```python
from build123d import *

# Parameters (mm, degrees)
SKETCH1_R           = 30.625
SKETCH1_R_2         = 12
BOSS_EXTRUDE1_DEPTH = 4.22
SKETCH1_4_R         = 52.5
SKETCH1_4_R_2       = 45
SKETCH1_4_R_3       = 30.625
BOSS_EXTRUDE2_DEPTH = 2
SKETCH2_R           = 1.5
CUT_EXTRUDE1_DEPTH  = 20


with BuildPart() as part:
    # Sketch1 → Boss-Extrude1 (new body)
    with BuildSketch(Plane.XY):
        Circle(SKETCH1_R)
        Circle(SKETCH1_R_2, mode=Mode.SUBTRACT)
    extrude(amount=-BOSS_EXTRUDE1_DEPTH)

    # Sketch1_4 → Boss-Extrude2 (add)
    # profile 1 of 2: a face of its own
    with BuildSketch(Plane.XY):
        Circle(SKETCH1_4_R)
        Circle(SKETCH1_4_R_2, mode=Mode.SUBTRACT)
    # profile 2 of 2: a face of its own
    with BuildSketch(Plane.XY):
        Circle(SKETCH1_4_R_2)
        Circle(SKETCH1_4_R_3, mode=Mode.SUBTRACT)
    extrude(amount=-BOSS_EXTRUDE2_DEPTH)

    # Sketch2 → Cut-Extrude1 (cut)
    with BuildSketch(Plane.XY):
        with Locations((-34.471455583, 34.471455583)):
            Circle(SKETCH2_R)
        with Locations((34.471455583, 34.471455583)):
            Circle(SKETCH2_R)
        with Locations((34.471455583, -34.471455583)):
            Circle(SKETCH2_R)
        with Locations((-34.471455583, -34.471455583)):
            Circle(SKETCH2_R)
        with Locations((0, 22.5)):
            Circle(SKETCH2_R)
        with Locations((22.5, 0)):
            Circle(SKETCH2_R)
        with Locations((0, -22.5)):
            Circle(SKETCH2_R)
        with Locations((-22.5, 0)):
            Circle(SKETCH2_R)
    extrude(amount=-CUT_EXTRUDE1_DEPTH, mode=Mode.SUBTRACT)


solid = part.part
```
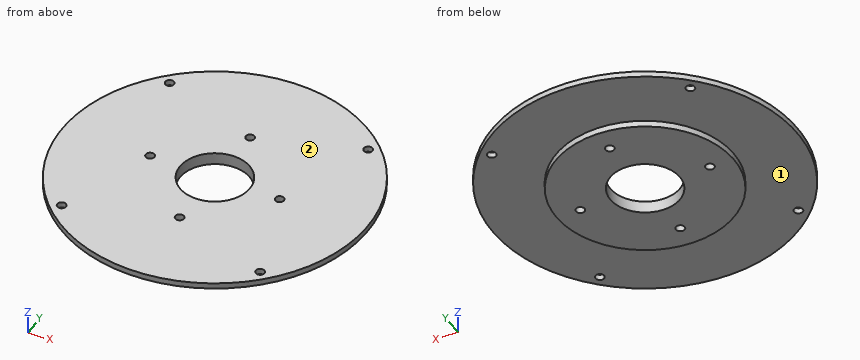
The model under review builds one solid part; all positions refer to its coordinate system, in mm. Face numbers are marked on the shaded views. A direction names the side the tool comes from. Round coordinates to 2 decimals unless told otherwise and drop trailing zeros. Order: outer loops, then holes, each group sorted by start corner. A loop starts at its lowest first (then second) coordinate and runs counter-clockwise, first axis right, second up.
(1) Take a section at C-C, the plane z = -3.3. State the section outline as (x, y) points (3 decimals).
Working result:
outline: circle Ø61.25 at (0, 0); hole circle Ø3 at (-22.5, 0); hole circle Ø24 at (0, 0); hole circle Ø3 at (0, -22.5); hole circle Ø3 at (0, 22.5); hole circle Ø3 at (22.5, 0)
(2) Take a section at A-A, the plane y = 0. State the section outline as (x, z) points (3 decimals), plus the area to 3 significant figures.
Working result:
outline: (-52.5, -2) - (-30.625, -2) - (-30.625, -4.22) - (-24, -4.22) - (-24, 0) - (-52.5, 0) - close; (-21, -4.22) - (-12, -4.22) - (-12, 0) - (-21, 0) - close; (12, -4.22) - (21, -4.22) - (21, 0) - (12, 0) - close; (24, -4.22) - (30.625, -4.22) - (30.625, -2) - (52.5, -2) - (52.5, 0) - (24, 0) - close
area: 219 mm2
(3) Take a section at D-D, the plane x = -22.5. State the section outline as (y, z) points, plus the area to 3 significant figures.
Working result:
outline: (-47.43, -2) - (-20.78, -2) - (-20.78, -4.22) - (-1.5, -4.22) - (-1.5, 0) - (-47.43, 0) - close; (1.5, -4.22) - (20.78, -4.22) - (20.78, -2) - (47.43, -2) - (47.43, 0) - (1.5, 0) - close
area: 269 mm2
(4) For P1, Ø4, axis at x = 34.47, y = 34.47, coming from the -Z side; P2, Ø1, axis at y = 5, z = -3.5, coming from the -X side, all flat-tipped, find the tip position at first contact; note any pin that passes through.
Working result:
P1: stops at z = -2
P2: stops at x = -30.29
(5) Tool access review of the marked faces 1 and 2: name each direction out of +Z, -Z, +X, -X, +Y, -Y from which nothing blocks a thin tool from reaching the whole face with its end or side.
Working result:
face 1: -Z
face 2: +Z, +X, -X, +Y, -Y
(6) Wall thickness on L1, parallel to Y at x = 0, z = -2.3 (3 decimals); L2, parallel to Z at x = 43.5, y = 4.5; L3, parallel to Y at x = 22.5, z = -2.05: over which ranges is each line inside the solid? List them lowest first.
Working result:
L1: y = -30.625 to -24, -21 to -12, 12 to 21, 24 to 30.625
L2: z = -2 to 0
L3: y = -20.78 to -1.5, 1.5 to 20.78
